The model under review builds one solid part; all positions refer to its coordinate system, in mm. Give positions to 0.01 mm unless a question says otherwise; leave off trailing zeros. Order: outer loops, then holes, each group sorted by start corner. A loop starts at its lowest first (then second) coordinate and runs counter-clockwise, first axis right, second up. Notation, with made-up numbers: M 38.25,69.5 L 45.25,69.5 A22 cw 45.25,77.5 Z; hole C 53,26 d7. An arc over 180 degrees is marked long. One line per question, with ' | ' between items. Start each with the question number.
1. Wall thickness on L1, parallel to Y at x = -34, z = 0.2; L2, parallel to Y at x = -32.5, z = 0.65; L3, parallel to X at y = -29.5, z = 0.75: over which ranges is each line inside the solid? List them lowest first.
2. We need section D-D on z = 0.4. Count the separate pieces of the cut face and the enclosed holes in it, then the cut area to 3 significant figures.
3. We need section C-C on x = -33.75. Write out the cut boundary in (y, z), then the cut area to 3 significant figures.
4. We need section A-A on y = -12.5. Write out the cut boundary in (x, z), then the cut area to 3 significant figures.
5. We need section B-B on x = 0. Write out the cut boundary in (y, z).
6. Insertion check: P1, Ø1, axis at x = -25, y = 26.5, coming from the -Z side; P2, Ø0.8, axis at x = -5, z = 0.5, coming from the +Y side. Each pin has a flat end and moves straight along its axis. Give the tip position at first contact, or say it passes through.
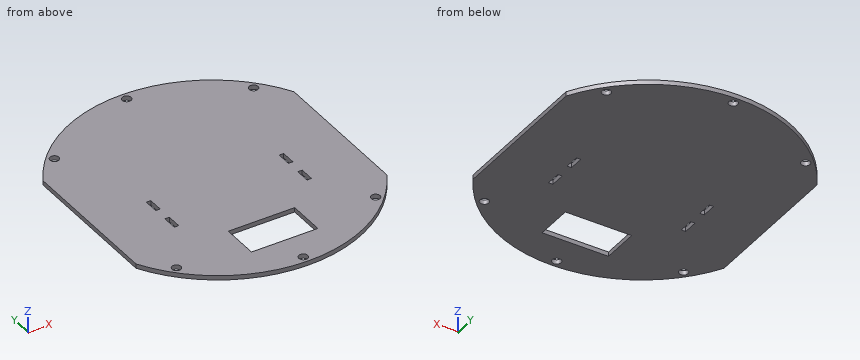
```python
from build123d import *

# Parameters (mm, degrees)
F0_R     = 1.5
F0_W     = 1.5
F0_H     = 5
F0_W_2   = 22.5
F0_H_2   = 12.5
F1_DEPTH = 1.5


with BuildPart() as f1:
    # F0 (on Top) → F1 (new body)
    with BuildSketch(Plane.XY):
        with BuildLine():
            Line((42.5, -25), (42.5, 25))
            ThreePointArc((42.5, 25), (0, 50), (-42.5, 25))
            Line((-42.5, 25), (-42.5, -25))
            ThreePointArc((-42.5, -25), (0, -50), (42.5, -25))
        make_face()
        with Locations((-33.75, -32.814674)):
            Circle(F0_R, mode=Mode.SUBTRACT)
        with Locations((-22.5, -12.5)):
            Rectangle(F0_W, F0_H, mode=Mode.SUBTRACT)
        with Locations((-22.5, -2.5)):
            Rectangle(F0_W, F0_H, mode=Mode.SUBTRACT)
        with Locations((0, -47.5)):
            Circle(F0_R, mode=Mode.SUBTRACT)
        with Locations((0, -31.25)):
            Rectangle(F0_W_2, F0_H_2, mode=Mode.SUBTRACT)
        with Locations((33.75, -32.814674)):
            Circle(F0_R, mode=Mode.SUBTRACT)
        with Locations((22.5, -12.5)):
            Rectangle(F0_W, F0_H, mode=Mode.SUBTRACT)
        with Locations((22.5, -2.5)):
            Rectangle(F0_W, F0_H, mode=Mode.SUBTRACT)
        with Locations((-33.75, 32.814674)):
            Circle(F0_R, mode=Mode.SUBTRACT)
        with Locations((0, 47.5)):
            Circle(F0_R, mode=Mode.SUBTRACT)
        with Locations((33.75, 32.814674)):
            Circle(F0_R, mode=Mode.SUBTRACT)
    extrude(amount=F1_DEPTH)


solid = f1.part
```
Entries:
1) L1: y = -36.14 to -34.29, -31.34 to 31.34, 34.29 to 36.14 | L2: y = -37.54 to -33.64, -31.99 to 31.99, 33.64 to 37.54 | L3: x = -39.67 to -11.25, 11.25 to 39.67
2) separate pieces: 1 | enclosed holes: 11 | area: 6,920 mm^2
3) outline: M -36.38,0 L -34.31,0 L -34.31,1.5 L -36.38,1.5 Z; M -31.31,0 L 31.31,0 L 31.31,1.5 L -31.31,1.5 Z; M 34.31,0 L 36.38,0 L 36.38,1.5 L 34.31,1.5 Z | area: 100 mm^2
4) outline: M -42.5,0 L -23.25,0 L -23.25,1.5 L -42.5,1.5 Z; M -21.75,0 L 21.75,0 L 21.75,1.5 L -21.75,1.5 Z; M 23.25,0 L 42.5,0 L 42.5,1.5 L 23.25,1.5 Z | area: 123 mm^2
5) outline: M -50,0 L -49,0 L -49,1.5 L -50,1.5 Z; M -46,0 L -37.5,0 L -37.5,1.5 L -46,1.5 Z; M -25,0 L 46,0 L 46,1.5 L -25,1.5 Z; M 49,0 L 50,0 L 50,1.5 L 49,1.5 Z
6) P1: stops at z = 0 | P2: stops at y = 49.78
